from build123d import *

# Parameters (mm, degrees)
SKETCH_W        = 150
SKETCH_H        = 120
PAD_DEPTH       = 60
SKETCH003_W     = 146
SKETCH003_H     = 116
POCKET_DEPTH    = 60
SKETCH004_R     = 6.5
POCKET001_DEPTH = 2
FILLET_R        = 1.9


with BuildPart() as part:
    # Sketch → Pad (new body)
    with BuildSketch(Plane.XY):
        with Locations((75, 60)):
            Rectangle(SKETCH_W, SKETCH_H)
    extrude(amount=PAD_DEPTH)

    # Sketch003 → Pocket (cut)
    with BuildSketch(Plane.XY):
        with Locations((75, 60)):
            Rectangle(SKETCH003_W, SKETCH003_H)
    extrude(amount=POCKET_DEPTH, mode=Mode.SUBTRACT)

    # Sketch004 → Pocket001 (cut)
    with BuildSketch(Plane.XZ.offset(-120)):
        with Locations((125, 30)):
            Circle(SKETCH004_R)
    extrude(amount=POCKET001_DEPTH, mode=Mode.SUBTRACT)

    # Fillet
    fillet_edges = [part.edges().sort_by_distance(p)[0] for p in [
        (150, 0, 30),
        (0, 0, 30),
        (0, 120, 30),
        (150, 120, 30),
    ]]
    fillet(fillet_edges, radius=FILLET_R)


solid = part.part
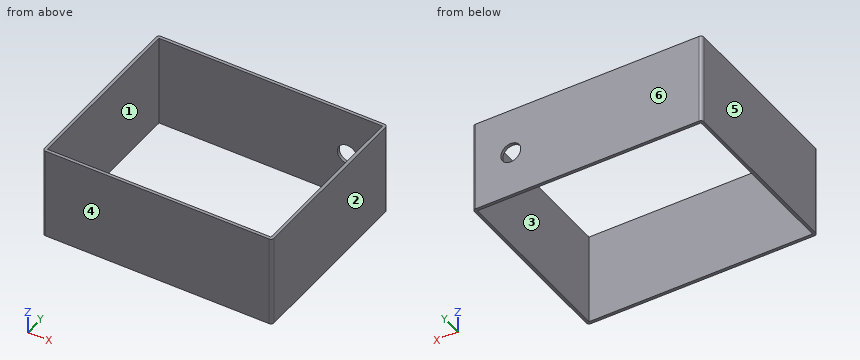
Geometry check sheet. Reference: the model listing, model coordinates, mm. Face numbers are marked on the shaded views. A direction names the side the tool comes from. Round coordinates to 2 decimals unless told otherwise and drop trailing zeros. Loops run counter-clockwise (first coordinate to the right, second up) from the corner with the lowest first, then second, coordinate; pieces in that order, holes last. Notation, with made-up numbers: (76.5, 70) -> (129.5, 70) arc R17 ccw to (129.5, 87) -> close; hole circle Ø10 at (-27.75, -12). An arc over 180 degrees is marked (long way). Answer as a JSON object with one key per item and string values. Group by question number.
Item 1: Cross-section at D-D, the plane z = 30. Record the cut outline in (x, y), plus the area to 3 significant figures.
Item 2: Depth check by flat-ended pin: pin 1 Ø11.5 at (x, z) = (125, 30) entering from +Y. Enter the tip coordinate at first touch or a pass-through.
Item 3: Thickness scan on line 1 along Y through (x, z) = (56, 5.5); line 2 along X through (y, z) = (55, 10); line 3 along Z through (x, y) = (125, 119). Record the ranges inside material, lowest first.
Item 4: Release check for a two-part mould opening along Y. For the marked faces 3, 4, 5 and 6 record: pulls with the +Y half, pulls with the -Y half, needs draft (parallel to the pull), parting line crosses it, or undercut.
Item 5: Cross-section at A-A, the plane y = 92. Record the cut outline in (x, z), plus the area to 3 significant figures.
Item 6: Set-up check for the marked faces 1 and 2: record each of +Z, -Z, +X, -X, +Y, -Y from which the full face is reachable in a straight line by a thin tool's end or side.
Item 7: Cross-section at B-B, the plane z = 51. Record the cut outline in (x, y).
Item 8: Cross-section at C-C, the plane x = 125. Record the cut outline in (y, z), plus the area to 3 significant figures.
Determined:
{
 "1": {"outline": "(0, 1.9) arc R1.9 ccw to (1.9, 0) -> (148.1, 0) arc R1.9 ccw to (150, 1.9) -> (150, 118.1) arc R1.9 ccw to (148.1, 120) -> (131.5, 120) -> (131.5, 118) -> (148, 118) -> (148, 2) -> (2, 2) -> (2, 118) -> (118.5, 118) -> (118.5, 120) -> (1.9, 120) arc R1.9 ccw to (0, 118.1) -> close", "area": "1,030 mm²"},
 "2": {"pin 1": "stops at y = 2"},
 "3": {"line 1": "y = 0 to 2, 118 to 120", "line 2": "x = 0 to 2, 148 to 150", "line 3": "z = 0 to 23.5, 36.5 to 60"},
 "4": {"face 3": "undercut", "face 4": "pulls with the -Y half", "face 5": "needs draft", "face 6": "pulls with the +Y half"},
 "5": {"outline": "(0, 0) -> (2, 0) -> (2, 60) -> (0, 60) -> close; (148, 0) -> (150, 0) -> (150, 60) -> (148, 60) -> close", "area": "240 mm²"},
 "6": {"face 1": "+Z, -Z", "face 2": "+Z, -Z, +X, +Y, -Y"},
 "7": {"outline": "(0, 1.9) arc R1.9 ccw to (1.9, 0) -> (148.1, 0) arc R1.9 ccw to (150, 1.9) -> (150, 118.1) arc R1.9 ccw to (148.1, 120) -> (1.9, 120) arc R1.9 ccw to (0, 118.1) -> close; hole (2, 2) -> (148, 2) -> (148, 118) -> (2, 118) -> close"},
 "8": {"outline": "(0, 0) -> (2, 0) -> (2, 60) -> (0, 60) -> close; (118, 0) -> (120, 0) -> (120, 23.5) -> (118, 23.5) -> close; (118, 36.5) -> (120, 36.5) -> (120, 60) -> (118, 60) -> close", "area": "214 mm²"}
}
